Source: CAD feature listing. Evaluate the final solid. Frame: model axes, mm. A direction names the side the tool comes from. Give positions to 0.01 mm unless a question says otherwise; leave off trailing zeros. Order: outer loops, then holes, each group sorted by start corner. A loop starts at its lowest first (then second) coordinate and runs counter-clockwise, first axis right, second up.
1) Section C-C, the plane x = 12.25. Return loops of the section in (y, z).
2) Section A-A, the plane z = 2.5. Return loops of the section in (x, y).
3) Access query for faces 5 (the face through (8, -8, 3)), 6 (the face through (7, -8, 9)), 7 (the face through (14, -8, 6)). Directions: +Z, -Z, +X, -X, +Y, -Y. A direction counts if a zero-diameter tool reaches every point of the face in a straight line with its end or side. Return the directions, or none.
4) Draft query along X for faces 1 (the face through (5, -8, 7)), 2 (the face through (17.508, -9.656, 3.042)), 3 (the face through (11.08, -0.14, 7.1)), 4 (the face through (10, 0, 4)). Return one class per face: released by +X, released by -X, zero draft, split by the parting line, or undercut.
5) Material intervals for line 1 (Z direction, x = 13.5, y = -7.5); line 2 (Y direction, x = 16, z = 2); line 3 (X direction, y = -6, z = 0.75), sorted ascending.
6) First-contact query: P1, Ø1, axis at x = 17.5, y = -2, coming from the +Z side; P2, Ø2, axis at x = 10, y = -14.5, coming from the -Z side; P3, Ø2.5, axis at x = 16, y = -8.5, coming from the +Z side; P4, Ø0.8, axis at x = 7, y = -11.5, coming from the -Z side. Flat tips, straight axial feed; report the tip coordinate or a pass-through.
7) Section B-B, the plane y = -8.5. Return loops of the section in (x, z).
```python
from build123d import *

# Parameters (mm, degrees)
F1_DEPTH = 17
F2_R     = 0.5
F3_R     = 1.9
F4_DEPTH = 25
F5_R     = 5
F6_R     = 0.5
F7_R     = 1
F8_R     = 0.49999


# Not quite as in the source:
# - a fillet or chamfer is up to 0.001 mm smaller than in the source, because OpenCascade refuses the exact size


with BuildPart() as f1:
    # F0 (on Front) → F1 (new body)
    with BuildSketch(Plane.XZ):
        with BuildLine():
            Line((-12, 0), (0, 0))
            Line((0, 0), (0, 5.58898558))
            ThreePointArc((0, 5.58898558), (0.1203833365, 5.8796166635), (0.41101442, 6))
            Line((0.41101442, 6), (3, 6))
            Line((3, 6), (3, 9))
            Line((3, 9), (-2, 9))
            Line((-2, 9), (-4, 6))
            Line((-4, 6), (-12, 6))
            Line((-12, 6), (-12, 0))
        make_face()
    extrude(amount=F1_DEPTH)

    # F2
    f2_edges = [f1.edges().sort_by_distance(p)[0] for p in [
        (3, -8.5, 9),
    ]]
    fillet(f2_edges, radius=F2_R)

    # F3 (on face) → F4 (cut)
    with BuildSketch(Plane.XY.offset(6)):
        with Locations((-8, -8.5)):
            Circle(F3_R)
    extrude(amount=-F4_DEPTH, mode=Mode.SUBTRACT)

    # F5
    f5_edges = [f1.edges().sort_by_distance(p)[0] for p in [
        (-12, -17, 3),
        (-12, 0, 3),
    ]]
    fillet(f5_edges, radius=F5_R)

    # F6
    f6_edges = [f1.edges().sort_by_distance(p)[0] for p in [
        (-10.535534, -15.535534, 6),
    ]]
    fillet(f6_edges, radius=F6_R)

    # F7
    f7_edges = [f1.edges().sort_by_distance(p)[0] for p in [
        (-2, -8.5, 9),
    ]]
    fillet(f7_edges, radius=F7_R)

    # F8 (radius 0.5 in the source; OpenCascade refuses exactly that, so slightly less here)
    f8_edges = [f1.edges().sort_by_distance(p)[0] for p in [
        (-3.148433, -17, 7.27735),
        (-3.148433, 0, 7.27735),
    ]]
    fillet(f8_edges, radius=F8_R)


with BuildPart() as f10_1:
    # F10: instance of F1
    add(f1.part.mirror(Plane(origin=(4, -8.5, 7.25), x_dir=(0, 1, 0), z_dir=(1, 0, 0))))


solid = f10_1.part
```
From the geometry:
1. outline: (-17, 0) - (0, 0) - (0, 5.5) arc R0.5 ccw to (-0.5, 6) - (-16.5, 6) arc R0.5 ccw to (-17, 5.5) - close
2. outline: (8, -17) - (15, -17) arc R5 ccw to (20, -12) - (20, -5) arc R5 ccw to (15, 0) - (8, 0) - close; hole circle Ø3.8 at (16, -8.5)
3. face 5: -Z, -X, +Y, -Y
3. face 6: +Z, +X, -X, +Y, -Y
3. face 7: +Z, +X, +Y, -Y
4. face 1: released by -X
4. face 2: undercut
4. face 3: released by +X
4. face 4: zero draft
5. line 1: z = 0 to 6
5. line 2: y = -16.9 to -10.4, -6.6 to -0.1
5. line 3: x = 8 to 20
6. P1: stops at z = 6
6. P2: stops at z = 0
6. P3: passes through
6. P4: stops at z = 6
7. outline: (5, 6) - (7.59, 6) arc R0.41 cw to (8, 5.59) - (8, 0) - (14.1, 0) - (14.1, 6) - (12, 6) - (10.3, 8.55) arc R1 ccw to (9.46, 9) - (5.5, 9) arc R0.5 ccw to (5, 8.5) - close; (17.9, 0) - (20, 0) - (20, 5.5) arc R0.5 ccw to (19.5, 6) - (17.9, 6) - close
